Read the model definition and answer for the solid it produces. Units are mm, in the model's axes. A direction names the side the tool comes from. Give positions to 0.01 mm unless a question says otherwise; leave off trailing zeros. Order: outer loops, then holes, each group sorted by start corner. A loop starts at its lowest first (then second) coordinate and runs counter-clockwise, first axis right, second up. Notation, with made-up numbers: (45, 22.25) - (75, 22.25) arc R21 ccw to (75, 36.25) - close; hole circle Ø8 at (-0.75, -30). An arc over 180 degrees is marked (long way). Write item = value, one per line.
```python
from build123d import *

# Parameters (mm, degrees)
SKETCH1_W           = 60
SKETCH1_H           = 84
RAIL_PLATE_DEPTH    = 6
DOVETAIL_RAIL_DEPTH = 80
SKETCH3_R           = 1.7
M3_HOLES_DEPTH      = 7
SKETCH4_R           = 3
COUNTERBORES_DEPTH  = 4


with BuildPart() as part:
    # Sketch1 → Rail Plate (new body)
    with BuildSketch(Plane(origin=(0, -34.4, 0), x_dir=(1, 0, 0), z_dir=(0, 1, 0))):
        with Locations((0, -70)):
            Rectangle(SKETCH1_W, SKETCH1_H)
    extrude(amount=RAIL_PLATE_DEPTH)

    # Sketch2 → Dovetail Rail (add)
    with BuildSketch(Plane.XY.offset(30)):
        Polygon((-15, -33.9), (15, -33.9), (19, -40.4), (-19, -40.4), align=None)
    extrude(amount=DOVETAIL_RAIL_DEPTH)

    # Sketch3 → M3 Holes (cut)
    with BuildSketch(Plane(origin=(0, -34.9, 0), x_dir=(1, 0, 0), z_dir=(0, 1, 0))):
        with Locations(Location((-22, -91, 0), (0, 0, 270))):
            Circle(SKETCH3_R)
        with Locations(Location((-22, -49, 0), (0, 0, 270))):
            Circle(SKETCH3_R)
        with Locations(Location((22, -91, 0), (0, 0, 270))):
            Circle(SKETCH3_R)
        with Locations(Location((22, -49, 0), (0, 0, 270))):
            Circle(SKETCH3_R)
    extrude(amount=M3_HOLES_DEPTH, mode=Mode.SUBTRACT)

    # Sketch4 → Counterbores (cut)
    with BuildSketch(Plane(origin=(0, -34.9, 0), x_dir=(1, 0, 0), z_dir=(0, 1, 0))):
        with Locations(Location((-22, -91, 0), (0, 0, 270))):
            Circle(SKETCH4_R)
        with Locations(Location((-22, -49, 0), (0, 0, 270))):
            Circle(SKETCH4_R)
        with Locations(Location((22, -91, 0), (0, 0, 270))):
            Circle(SKETCH4_R)
        with Locations(Location((22, -49, 0), (0, 0, 270))):
            Circle(SKETCH4_R)
    extrude(amount=COUNTERBORES_DEPTH, mode=Mode.SUBTRACT)


solid = part.part
```
1. Determine the mould class of faces 6 (the face through (0, -31, 112)), 7 (the face through (17.13, -37.36, 69.44)), 8 (the face through (0, -28.4, 69)), 9 (the face through (-22, -30.9, 51)) for opening direction Y: +Y half, -Y half, draft (parallel to the pull), parting line (faces both ways), or undercut.
Recorded:
face_6 = draft
face_7 = undercut
face_8 = +Y half
face_9 = -Y half
2. Section A-A (x = -22) is taken. Determine the outline of the cut face in (y, z).
Recorded:
outline = (-34.4, 28) - (-28.4, 28) - (-28.4, 47.3) - (-30.9, 47.3) - (-30.9, 46) - (-34.4, 46) - close; (-34.4, 52) - (-30.9, 52) - (-30.9, 50.7) - (-28.4, 50.7) - (-28.4, 89.3) - (-30.9, 89.3) - (-30.9, 88) - (-34.4, 88) - close; (-34.4, 94) - (-30.9, 94) - (-30.9, 92.7) - (-28.4, 92.7) - (-28.4, 112) - (-34.4, 112) - close
3. Section C-C (x = -6) is taken. Determine the outline of the cut face in (y, z).
Recorded:
outline = (-40.4, 30) - (-34.4, 30) - (-34.4, 28) - (-28.4, 28) - (-28.4, 112) - (-34.4, 112) - (-34.4, 110) - (-40.4, 110) - close
4. Section B-B (z = 49) is taken. Determine the outline of the cut face in (x, y), and give its area (3 significant figures).
Recorded:
outline = (-30, -34.4) - (-25, -34.4) - (-25, -30.9) - (-23.7, -30.9) - (-23.7, -28.4) - (-30, -28.4) - close; (-20.3, -30.9) - (-19, -30.9) - (-19, -34.4) - (-15.31, -34.4) - (-19, -40.4) - (19, -40.4) - (15.31, -34.4) - (19, -34.4) - (19, -30.9) - (20.3, -30.9) - (20.3, -28.4) - (-20.3, -28.4) - close; (23.7, -30.9) - (25, -30.9) - (25, -34.4) - (30, -34.4) - (30, -28.4) - (23.7, -28.4) - close
area = 507 mm^2
5. Straight lines are drawn through the part: L1, parallel to Z at x = -22, y = -33.1; L2, parallel to X at y = -32.65, z = 91; L3, parallel to Z at x = 22, y = -28.95. For each, find the intervals that lie inside material, in ascending order. Write a range as [from, to].
Recorded:
L1 = [28, 46], [52, 88], [94, 112]
L2 = [-30, -25], [-19, 19], [25, 30]
L3 = [28, 47.3], [50.7, 89.3], [92.7, 112]
6. For faces 1 (the face through (0, -37, 30)), 2 (the face through (23.15, -29.67, 47.75)), 3 (the face through (0, -40.4, 69)), 4 (the face through (-22, -33, 88)), 5 (the face through (0, -37, 110)), determine the directions among +Z, -Z, +X, -X, +Y, -Y from which every point of the face is accessible in a straight line to the end or side of a thin tool.
Recorded:
face_1 = -Z, +X, -X, -Y
face_2 = +Y, -Y
face_3 = +Z, -Z, +X, -X, -Y
face_4 = -Y
face_5 = +Z, +X, -X, -Y
7. Flat-ended cylindrical pins translate along their axes: pin 1 (2 mm diameter, centred on x = -22, z = 49, fed in from +Y); pin 2 (6.5 mm diameter, centred on x = -21, z = 47.5, fed in from -Y); pin 3 (5 mm diameter, centred on x = 23, z = 91, fed in from -Y); pin 4 (5 mm diameter, centred on x = -4, y = -38, fed in from +Z). Find the tip coordinate at first contact, or state that the pin passes through.
Recorded:
pin_1 = through
pin_2 = -40.4
pin_3 = -34.4
pin_4 = 110
8. Section D-D (x = 17) is taken. Determine the outline of the cut face in (y, z).
Recorded:
outline = (-40.4, 30) - (-37.15, 30) - (-37.15, 110) - (-40.4, 110) - close; (-34.4, 28) - (-28.4, 28) - (-28.4, 112) - (-34.4, 112) - close
